Source: three-view drawing plus pictorial views. Frame: mm from the lowest corner of the part. A direction names the side the tool comes from. Give positions to 0.01 mm unless a question says otherwise; leave off trailing zeros. Order: outer loops, then holes, each group sorted by start corner. A loop starts at its lowest first (then second) coordinate and runs counter-clockwise, first axis right, second up.
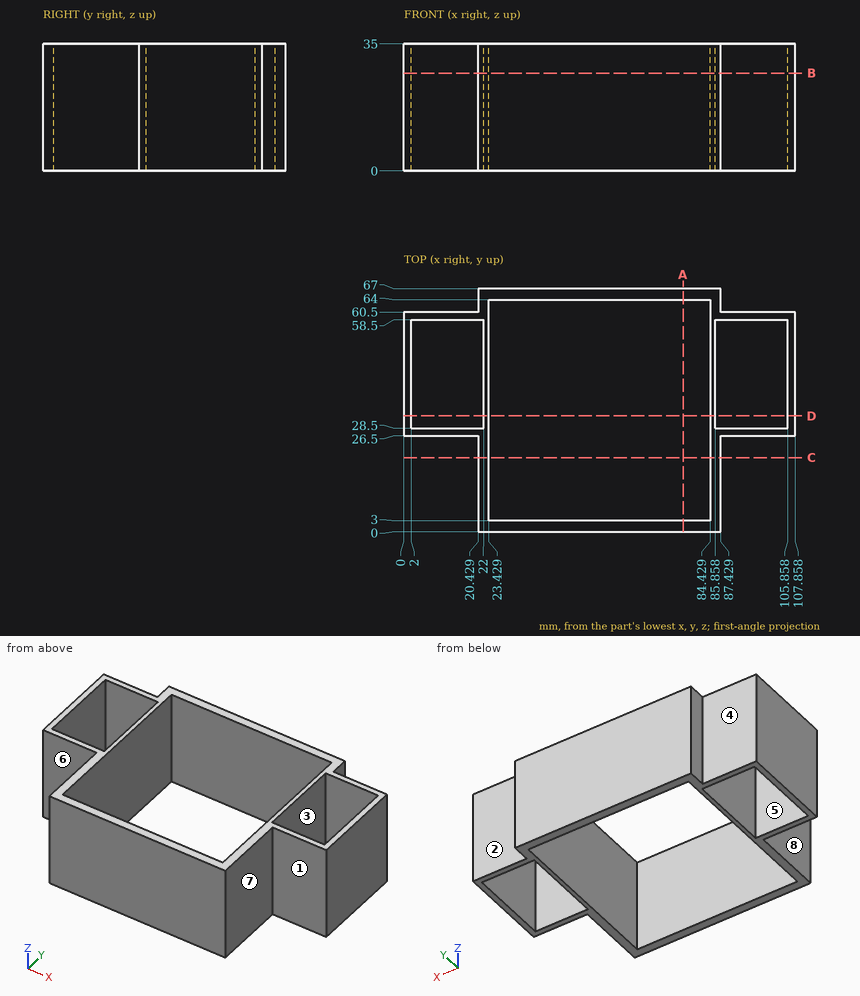
(1) Line query: line 1 along X through (y, z) = (29, 5); line 2 along Y through (x, z) = (31, 19); line 3 along Y through (x, z) = (17, 6). Output: solid intervals per line, ascending.
(2) Section A-A, the plane x = 77. Return loops of the section in (y, z), plus the area to 3 significant figures.
(3) Pin query (flat end, axial travel): pin 1 Ø5 at (x, y) = (84.5, 19.5) entering from -Z; pin 2 Ø13 at (y, z) = (11.5, 26) entering from +X; pin 3 Ø16.5 at (x, z) = (98, 19.5) entering from +Y; pin 4 Ø16.5 at (x, z) = (101, 10.5) entering from -Y. Return the tip coordinate at first contact, or that it passes through.
(4) Section C-C, the plane y = 20.5. Return loops of the section in (x, z).
(5) Section B-B, the plane z = 27. Return loops of the section in (x, y), plus the area to 3 significant figures.
(6) Draft query along X for the marked faces 5, 6, 7 and 8. Return one class per face: +X half, -X half, draft (parallel to the pull), parting line (faces both ways), or undercut.
(7) Section D-D, the plane y = 32. Return loops of the section in (x, z).
(8) Access query for the marked faces 1, 2, 3 and 4. Directions: +Z, -Z, +X, -X, +Y, -Y. A direction counts if a zero-diameter tool reaches every point of the face in a straight line with its end or side. Return the directions, or none.
Checks:
1. line 1: x = 0 to 2, 22 to 23.43, 84.43 to 85.86, 105.86 to 107.86
1. line 2: y = 0 to 3, 64 to 67
1. line 3: y = 26.5 to 28.5, 58.5 to 60.5
2. outline: (0, 0) - (3, 0) - (3, 35) - (0, 35) - close; (64, 0) - (67, 0) - (67, 35) - (64, 35) - close
2. area: 210 mm2
3. pin 1: stops at z = 0
3. pin 2: stops at x = 87.43
3. pin 3: stops at y = 60.5
3. pin 4: stops at y = 26.5
4. outline: (20.43, 0) - (23.43, 0) - (23.43, 35) - (20.43, 35) - close; (84.43, 0) - (87.43, 0) - (87.43, 35) - (84.43, 35) - close
5. outline: (0, 26.5) - (20.43, 26.5) - (20.43, 0) - (87.43, 0) - (87.43, 26.5) - (107.86, 26.5) - (107.86, 60.5) - (87.43, 60.5) - (87.43, 67) - (20.43, 67) - (20.43, 60.5) - (0, 60.5) - close; hole (2, 28.5) - (22, 28.5) - (22, 58.5) - (2, 58.5) - close; hole (23.43, 3) - (84.43, 3) - (84.43, 64) - (23.43, 64) - close; hole (85.86, 28.5) - (105.86, 28.5) - (105.86, 58.5) - (85.86, 58.5) - close
5. area: 957 mm2
6. face 5: undercut
6. face 6: draft
6. face 7: +X half
6. face 8: -X half
7. outline: (0, 0) - (2, 0) - (2, 35) - (0, 35) - close; (22, 0) - (23.43, 0) - (23.43, 35) - (22, 35) - close; (84.43, 0) - (85.86, 0) - (85.86, 35) - (84.43, 35) - close; (105.86, 0) - (107.86, 0) - (107.86, 35) - (105.86, 35) - close
8. face 1: +Z, -Z, +X, -Y
8. face 2: +Z, -Z, +X, +Y
8. face 3: +Z, -Z
8. face 4: +Z, -Z, -X, +Y
